The figure shows three views and two pictorial views of one solid part (mm, origin at its lowest corner). Answer the questions. Coordinates: 2 decimals unless noted, no trailing zeros. Loops run counter-clockwise (first coordinate to the right, second up) from the corner with the lowest first, then second, coordinate; pieces in that order, holes last.
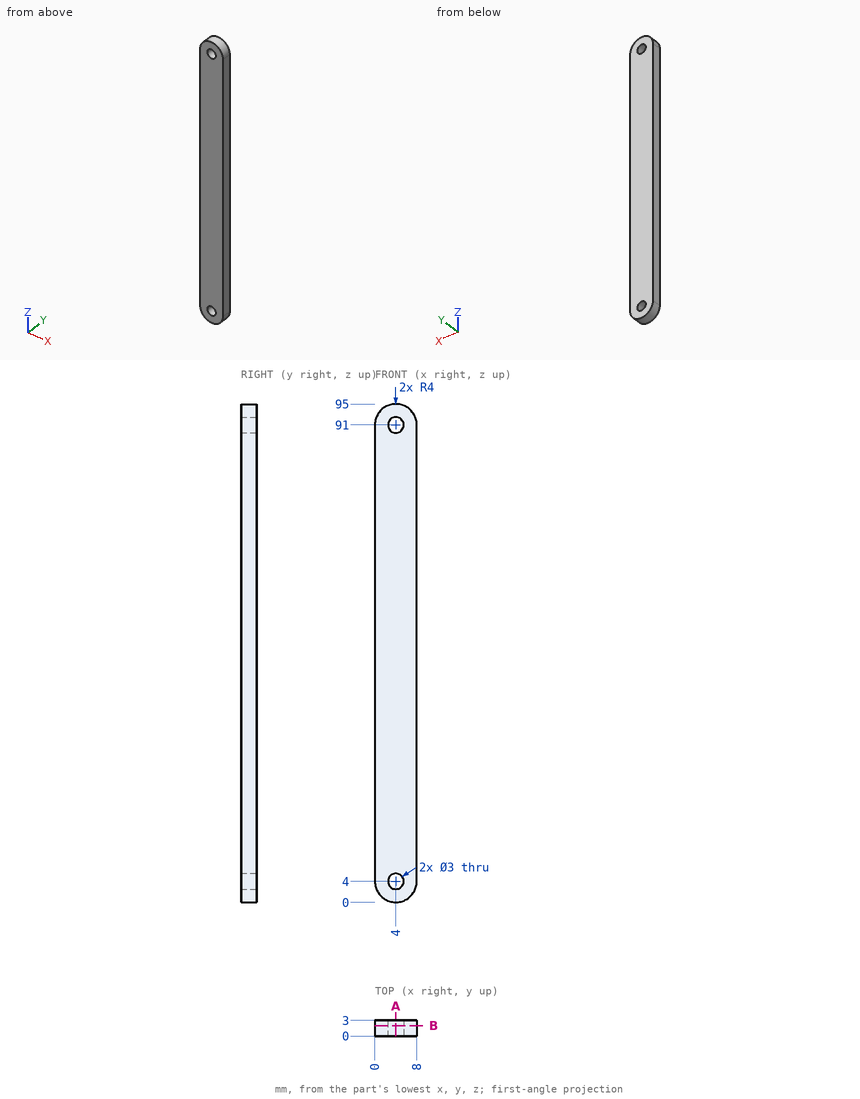
1. This flat-tipped pin is pushed along its axis until it touches: P1, Ø2.5, axis at x = 4, z = 4, coming from the -Y side. Where does it stop, or does it pass through?
2. A cutting plane is placed at A-A, the plane x = 4. Give the vertices of the cut face in (y, z).
3. Straight lines are drawn through the part: probe 1 along Z at (x, y) = (4, 1.3); probe 2 along X at (y, z) = (1.8, 4); probe 3 along Z at (x, y) = (5, 1.1). For each, find the intervals that lie inside material, in ascending order.
4. A cutting plane is placed at B-B, the plane y = 2. Give the vertices of the cut face in (x, z), then the cut area to 3 significant figures.
Answers below:
1. P1: passes through
2. outline: (0, 0) - (3, 0) - (3, 2.5) - (0, 2.5) - close; (0, 5.5) - (3, 5.5) - (3, 89.5) - (0, 89.5) - close; (0, 92.5) - (3, 92.5) - (3, 95) - (0, 95) - close
3. probe 1: z = 0 to 2.5, 5.5 to 89.5, 92.5 to 95
3. probe 2: x = 0 to 2.5, 5.5 to 8
3. probe 3: z = 0.13 to 2.88, 5.12 to 89.88, 92.12 to 94.87
4. outline: (0, 4) arc R4 ccw to (8, 4) - (8, 91) arc R4 ccw to (0, 91) - close; hole circle Ø3 at (4, 4); hole circle Ø3 at (4, 91)
4. area: 732 mm2
